Geometry: final body of the model. Coordinates: model frame, mm. A direction names the side the tool comes from. Give positions to 0.01 mm unless a question says otherwise; leave off trailing zeros. Write each loop counter-clockwise with the first axis right and the second up, starting at its lowest first coordinate (ties: lowest second). Pieces come first, ordered by that corner, then holes. Notation, with made-up numbers: M 85,87.25 L 98,87.25 A37 ccw 98,125.25 Z; hole C 30,72.25 d6. An arc over 180 degrees is marked long. Use one line per item in the form item = value. Start each with the question number.
Item 1: Section query A-A on z = 3. Return loops of the section in (x, y), then the cut area to 3 significant figures.
Item 2: Section query C-C on x = -5. Return loops of the section in (y, z).
Item 3: Material intervals for line 1 along Z through (x, y) = (-10, 30); line 2 along X through (y, z) = (8.5, -1.25); line 3 along Y through (x, z) = (-3.75, 0.5), sorted ascending. Write a range as from..to.
Item 4: Section query B-B on z = 0.25. Return loops of the section in (x, y), then the cut area to 3 significant figures.
Item 5: Contact query for flat-ended pins moving along their axis: P1, Ø4, axis at x = -7, y = 24.5, coming from the -Z side; P2, Ø0.6, axis at y = 0, z = 3.5, coming from the -X side; P3, Ø0.9, axis at y = 2, z = 0, coming from the +X side; P4, Ø1, axis at x = -6.5, z = -1.5, coming from the +Y side. Output: stop coordinate, or through.
Item 6: Access query for faces 4 (the flat face through (-8.063, 21, 0)), 5 (the flat face through (0, 0.7, 4)), 6 (the cylindrical face through (-7.6, 0.3, 4.8)), 7 (the flat face through (0.537, 1, 0)). Directions: +Z, -Z, +X, -X, +Y, -Y. A direction counts if a zero-diameter tool reaches every point of the face in a straight line with its end or side. Return the directions, or none.
Item 7: Pull-direction query (Z, two-part tool) for faces 1 (the flat face through (-4, 3, 0)), 2 (the cylindrical face through (-0.075, 0.345, 5.732)), 3 (the flat face through (-8.3, 16.9, -2.567)); classes: released by +Z, released by -Z, zero draft, split by the parting line, or undercut.
Item 8: Section query D-D on y = 16.5. Return loops of the section in (x, z), then the cut area to 3 significant figures.
Autodesk Inventor part; units mm, degrees
ref_plane "YZ Plane" through (0, 0, 0) normal (1, 0, 0) x (0, 1, 0)
ref_plane "XZ Plane" through (0, 0, 0) normal (0, 1, 0) x (-1, 0, 0)
ref_plane "XY Plane" through (0, 0, 0) normal (0, 0, 1) x (1, 0, 0)
sketch "Sketch1" plane through (0, 0, 0) normal (0, 1, 0) x (-1, 0, 0)
  line L0 (-0.537, 0.033) -> (-0.537, -0.967)
  line L1 (-0.537, -0.467) -> (-0.537, -2.567)
  line L2 (-0.537, -2.567) -> (10.563, -2.567)
  line L3 (-0.537, -0.967) -> (-0.537, 0.033)
  line L4 (-0.537, 1.633) -> (10.563, 1.633)
  line L5 (-0.537, -0.467) -> (-0.537, 1.633)
  line L6 (10.563, 1.633) -> (10.563, -2.567)
  line L7 (10.563, 1.633) -> (8.063, 1.633)
  line L8 (8.063, 1.633) -> (8.063, -2.567)
  line L9 (10.563, -2.567) -> (10.563, 1.633)
  line L10 (7.7848, 1.633) -> (6.7848, 1.633)
  line L11 (6.7848, 1.633) -> (6.7848, 3.5399)
  line L12 (6.7848, 3.633) -> (7.2848, 3.633)
  line L13 (7.7848, 3.5399) -> (7.7848, 1.633)
  line L14 (0.4848, 1.633) -> (-0.5152, 1.633)
  line L15 (-0.5152, 1.633) -> (-0.5152, 4.1811)
  line L16 (-0.5152, 4.233) -> (0.0393, 4.233)
  line L17 (0.4848, 4.1049) -> (0.4848, 1.633)
  circle A0 centre (7.2848, 4.258) radius 0.625
  arc A1 (7.7848, 3.5399) -> (6.7848, 3.5399) centre (7.2848, 4.258) ccw
  circle A2 centre (0.0393, 4.858) radius 0.625
  arc A3 (0.4848, 4.1049) -> (-0.5152, 4.1811) centre (0.0393, 4.858) ccw
  point P0 (1.1114, -1.7636)
  point P1 (1.1114, -2.7636)
  point P2 (-0.0152, 4.233)
  point P3 (0.0393, 4.0356)
  point P4 (6.7848, 1.633)
  point P5 (-0.5152, 1.633)
  point P6 (7.2848, 1.633)
  dimension "d13" = 1.25
  dimension "d15" = 1.25
  dimension "d4" = 11.1
  dimension "d5" = 4.2
  dimension "d6" = 2.5
  dimension "d9" = 7.3
  dimension "d11" = 1
  dimension "d12" = 1
  dimension "d14" = 1.75
  dimension "d16" = 1.75
  dimension "d17" = 0.6
  dimension "d26" = 2
extrude "Extrusion1" add sketch "Sketch1" along normal blind 0.7 contours L11 A1 L13 L4
extrude "Extrusion2" add sketch "Sketch1" along normal blind 40 contours L8 L4 L6 L2
extrude "Extrusion3" add sketch "Sketch1" along normal blind 3 contours L5 L4 L8 L2 L1 L0
extrude "Extrusion4" add sketch "Sketch1" along normal blind 0.7 contours L15 A3 L17 L4
properties part number "optrode_holder_maelle"
Answer sheet:
q1.outline = M -7.78,0 L -6.78,0 L -6.78,0.7 L -7.78,0.7 Z; M -0.48,0 L 0.52,0 L 0.52,0.7 L -0.48,0.7 Z
q1.area = 1.40 mm2
q2.outline = M 0,-2.57 L 3,-2.57 L 3,1.63 L 0,1.63 Z
q3.line_1 = -2.57..1.63
q3.line_2 = -10.56..-8.06
q3.line_3 = 0..3
q4.outline = M -10.56,0 L 0.54,0 L 0.54,3 L -8.06,3 L -8.06,40 L -10.56,40 Z
q4.area = 126 mm2
q5.P1 = -2.57
q5.P2 = -8.03
q5.P3 = 0.54
q5.P4 = 3
q6.face_4 = +Z, -Z, +X, +Y
q6.face_5 = +Z, +X, -X, +Y
q6.face_6 = +Y, -Y
q6.face_7 = -Z, +X, +Y, -Y
q7.face_1 = zero draft
q7.face_2 = undercut
q7.face_3 = released by -Z
q8.outline = M -10.56,-2.57 L -8.06,-2.57 L -8.06,1.63 L -10.56,1.63 Z
q8.area = 10.5 mm2
